```python
from build123d import *

# Parameters (mm, degrees)
SKETCH1_W                      = 40
SKETCH1_H                      = 40
BOSS_EXTRUDE1_DEPTH            = 40
BOSS_EXTRUDE1_TAPER            = 7.125
SKETCH2_R                      = 30
BOSS_EXTRUDE2_DEPTH            = 25
BOSS_EXTRUDE3_REACH            = 152.083
BOSS_EXTRUDE3_END_RADIUS       = 30
SKETCH3_R                      = 15
BOSS_EXTRUDE4_START            = -5
SKETCH4_R                      = 8
BOSS_EXTRUDE4_DEPTH            = 12
BOSS_EXTRUDE5_START            = 5
SKETCH5_R                      = 8
BOSS_EXTRUDE5_DEPTH            = 10
CUT_EXTRUDE1_REACH             = 168
SKETCH8_R                      = 10
CUT_EXTRUDE1_DIRECTION_2_DEPTH = 100
HOLE1_D                        = 30


with BuildPart() as part:
    # Sketch1 → Boss-Extrude1 (new body)
    with BuildSketch(Plane(origin=(0, 0, 0), x_dir=(1, 0, 0), z_dir=(0, 1, 0))):
        Rectangle(SKETCH1_W, SKETCH1_H)
    extrude(amount=BOSS_EXTRUDE1_DEPTH, taper=BOSS_EXTRUDE1_TAPER)



with BuildPart() as body_2:
    # Sketch2 → Boss-Extrude2 (new, symmetric)
    with BuildSketch(Plane(origin=(0, 20, 0), x_dir=(1, 0, 0), z_dir=(0, 1, 0))):
        with Locations(Location((0, 110, 0), (0, 0, 270))):
            Circle(SKETCH2_R)
    extrude(amount=BOSS_EXTRUDE2_DEPTH, both=True)


with BuildPart() as part_1:
    add(part.part)

    add(body_2.part)  # Boss-Extrude3 merges body 2
    # Boss-Extrude3: up to this cylinder (the profile starts outside it)
    boss_extrude3_end = Plane(origin=(0, 20, -110), z_dir=(0, -1, 0)) * Cylinder(BOSS_EXTRUDE3_END_RADIUS, 365.166, mode=Mode.PRIVATE)
    # Sketch3 → Boss-Extrude3 (add, up to the surface)
    with BuildSketch(Plane.XY, mode=Mode.PRIVATE) as boss_extrude3_sk1:
        with Locations((0, 20)):
            Circle(SKETCH3_R)
    boss_extrude3_tool1 = extrude(boss_extrude3_sk1.sketch, amount=-BOSS_EXTRUDE3_REACH, mode=Mode.PRIVATE) - boss_extrude3_end
    add(boss_extrude3_tool1.solids().sort_by_distance((0, 20, 0))[0])

    # Sketch4 → Boss-Extrude4 (add)
    with BuildSketch(Plane(origin=(0, 0, 0), x_dir=(0, 0, -1), z_dir=(1, 0, 0)).offset(BOSS_EXTRUDE4_START)):
        with BuildLine():
            Line((20, 64), (20, 20))
            Line((20, 20), (60, 20))
            Line((60, 20), (60, 64))
            ThreePointArc((60, 64), (40, 84), (20, 64))
        make_face()
        with Locations((40, 64)):
            Circle(SKETCH4_R, mode=Mode.SUBTRACT)
    extrude(amount=BOSS_EXTRUDE4_DEPTH)

    # Sketch5 → Boss-Extrude5 (add)
    with BuildSketch(Plane(origin=(0, 0, 0), x_dir=(0, 0, -1), z_dir=(1, 0, 0)).offset(BOSS_EXTRUDE5_START)):
        with BuildLine():
            Line((-20, 0), (20, 0))
            Line((20, 0), (14.738148017, -27.790518414))
            ThreePointArc((14.738148017, -27.790518414), (0, -40), (-14.738148017, -27.790518414))
            Line((-14.738148017, -27.790518414), (-20, 0))
        make_face()
        with Locations((0, -25)):
            Circle(SKETCH5_R, mode=Mode.SUBTRACT)
    boss_extrude5 = extrude(amount=BOSS_EXTRUDE5_DEPTH)

    # Mirror1: Boss-Extrude5 across plane
    add(boss_extrude5.mirror(Plane(origin=(0, 0, 0), x_dir=(0, 0, 1), z_dir=(1, 0, 0))))

    # Cut-Extrude1: up to this plane
    cut_extrude1_end = Plane(origin=(-20, 0, 20), z_dir=(0, 0.1240344514504856, 0.9922779121059669))
    # Sketch8 → Cut-Extrude1 (cut, up to the surface)
    with BuildSketch(Plane.XY, mode=Mode.PRIVATE) as cut_extrude1_sk1:
        with Locations((0, 20)):
            Circle(SKETCH8_R)
    cut_extrude1_tool1 = split(extrude(cut_extrude1_sk1.sketch, amount=CUT_EXTRUDE1_REACH, mode=Mode.PRIVATE), bisect_by=cut_extrude1_end, keep=Keep.BOTH, mode=Mode.PRIVATE)
    add(cut_extrude1_tool1.solids().sort_by_distance((0, 20, 0))[0], mode=Mode.SUBTRACT)

    # Sketch8 → Cut-Extrude1 direction 2 (cut)
    with BuildSketch(Plane.XY):
        with Locations((0, 20)):
            Circle(SKETCH8_R)
    extrude(amount=-CUT_EXTRUDE1_DIRECTION_2_DEPTH, mode=Mode.SUBTRACT)

    # Hole1 (through all)
    with Locations(Plane(origin=(0, 45, 0), x_dir=(1, 0, 0), z_dir=(0, 1, 0))):
        with Locations((0, 110)):
            Hole(HOLE1_D / 2)


solid = part_1.part
```
The listing builds one solid part. Answer for the finished solid, in the listing's coordinates (mm). A direction names the side the tool comes from. Give positions to 0.01 mm unless a question says otherwise; leave off trailing zeros. Order: outer loops, then holes, each group sorted by start corner. A loop starts at its lowest first (then second) coordinate and runs counter-clockwise, first axis right, second up. Notation, with made-up numbers: (74.5, -6.75) -> (80.5, -6.75) arc R28 ccw to (80.5, 24.25) -> close; hole circle Ø8 at (63, 84). An arc over 180 degrees is marked (long way). One line per item, written item: value.
1) A tool of negligible diameter and unlimited length cuts with its end or side. For faces 1 (the flat face through (-9.93, -13.701, -17.406)), 2 (the cylindrical face through (-3.252, 5.357, -49.344)), 3 (the flat face through (-18, 0, 0)), 4 (the flat face through (-5, -15, 0)), 5 (the flat face through (14, -5, -104)), from which of +Z, -Z, +X, -X, +Y, -Y can it reach the whole face along a straight path? Write none if from no direction.
Reported:
face 1: +X, -X, -Y
face 2: none
face 3: +Z, -X, -Y
face 4: +Z, -Y
face 5: -Z, +X, -X, -Y
2) Determine the mould class of faces 6 (the cylindrical face through (1, 84, -40)), 7 (the flat face through (17, 0, 0)), 8 (the flat face through (-5, 54, -40)) for opening direction Z: pulls with the +Z half, pulls with the -Z half, needs draft (parallel to the pull), parting line crosses it, or undercut.
Reported:
face 6: parting line crosses it
face 7: needs draft
face 8: undercut
3) Find the intervals of material crossed by line 1 (Z direction, x = -7, y = -4); line 2 (Y direction, x = 0, z = -41); line 3 (X direction, y = -22.5, z = -15), in increasing order.
Reported:
line 1: z = -139.17 to -123.27, -96.73 to -80.83, -19.24 to 19.24
line 2: y = 5 to 10, 30 to 56.06, 71.94 to 83.97
line 3: x = -15 to -5, 5 to 15
4) Find section C-C, the plane y = 70. Determine the outline of the cut face in (x, z).
Reported:
outline: (-5, -59.08) -> (7, -59.08) -> (7, -45.29) -> (-5, -45.29) -> close; (-5, -34.71) -> (7, -34.71) -> (7, -20.92) -> (-5, -20.92) -> close
5) Flat-ended cylindrical pins translate along their axes: P1, Ø20, axis at y = 61.5, z = -34, coming from the -X side; P2, Ø20, axis at y = 59.5, z = -47.5, coming from the +X side; P3, Ø3.5, axis at x = -1.5, y = 52, coming from the -Z side. Find the tip coordinate at first contact, or state that the pin passes through.
Reported:
P1: stops at x = -5
P2: stops at x = 7
P3: stops at z = -60
6) Find section A-A, the plane z = -40. Determine the outline of the cut face in (x, y), plus the area to 3 significant figures.
Reported:
outline: (-5, 34.14) arc R15 ccw (long way) to (7, 33.27) -> (7, 56) -> (-5, 56) -> close; (-5, 72) -> (7, 72) -> (7, 84) -> (-5, 84) -> close; hole circle Ø20 at (0, 20)
area: 794 mm^2
7) Find section D-D, the plane z = 0. Count the separate pieces of the cut face and the enclosed holes in it, plus the area to 3 significant figures.
Reported:
separate pieces: 3
enclosed holes: 1
area: 1,570 mm^2
8) Find section B-B, the plane z = -110. Determine the outline of the cut face in (x, y).
Reported:
outline: (-30, -5) -> (-15, -5) -> (-15, 45) -> (-30, 45) -> close; (15, -5) -> (30, -5) -> (30, 45) -> (15, 45) -> close
